```python
from build123d import *

# Parameters (mm, degrees)
SKETCH1_R           = 4
SKETCH1_R_2         = 2.5
BOSS_EXTRUDE1_DEPTH = 5
BOSS_EXTRUDE2_START = 3.5
SKETCH2_R           = 12.5
SKETCH2_R_2         = 2.5
BOSS_EXTRUDE2_DEPTH = 3.5
CIRPATTERN1_COUNT   = 4
CIRPATTERN2_COUNT   = 4
CHAMFER1_SIZE       = 0.5
SKETCH9_R           = 2.5
BOSS_EXTRUDE3_DEPTH = 2.9


with BuildPart() as part:
    # Sketch1 → Boss-Extrude1 (new body)
    with BuildSketch(Plane.XY):
        Circle(SKETCH1_R)
        Circle(SKETCH1_R_2, mode=Mode.SUBTRACT)
    extrude(amount=-BOSS_EXTRUDE1_DEPTH)

    # Sketch2 → Boss-Extrude2 (add)
    with BuildSketch(Plane.XY.offset(BOSS_EXTRUDE2_START)):
        Circle(SKETCH2_R)
        Circle(SKETCH2_R_2, mode=Mode.SUBTRACT)
    extrude(amount=-BOSS_EXTRUDE2_DEPTH)

    # Sketch6 → Tap Drill for M3 Tap1 (revolve, cut)
    with BuildSketch(Plane(origin=(4, 0, -2.5), x_dir=(0, 0, -1), z_dir=(0, 1, 0))):
        Polygon((0, 0), (0, 5.751075774), (1.25, 5), (1.25, 0.025), (1.275, 0), align=None)
    tap_drill_for_m3_tap1 = revolve(axis=Axis((10.35, 0, -2.5), (-1, 0, 0)), mode=Mode.SUBTRACT)

    # Sketch8 → Tap Drill for M3 Tap2 (revolve, cut)
    with BuildSketch(Plane(origin=(-9, 0, 3.5), x_dir=(0, -1, 0), z_dir=(1, 0, 0))):
        Polygon((0, 0), (0, 5.751075774), (1.25, 5), (1.25, 0.025), (1.275, 0), align=None)
    tap_drill_for_m3_tap2 = revolve(axis=Axis((-9, 0, 9.85), (0, 0, -1)), mode=Mode.SUBTRACT)

    # CirPattern1: Tap Drill for M3 Tap2 ×4 about axis
    cirpattern1_axis = Axis((0, 0, 0), (0, 0, 1))
    for i in range(1, CIRPATTERN1_COUNT):
        add(tap_drill_for_m3_tap2.rotate(cirpattern1_axis, i * 360 / CIRPATTERN1_COUNT), mode=Mode.SUBTRACT)

    # CirPattern2: Tap Drill for M3 Tap1 ×4 about axis
    cirpattern2_axis = Axis((0, 0, 0), (0, 0, 1))
    for i in range(1, CIRPATTERN2_COUNT):
        add(tap_drill_for_m3_tap1.rotate(cirpattern2_axis, i * 360 / CIRPATTERN2_COUNT), mode=Mode.SUBTRACT)

    # Chamfer1
    chamfer1_edges = [part.edges().sort_by_distance(p)[0] for p in [
        (-4, 0, -5),
    ]]
    chamfer(chamfer1_edges, length=CHAMFER1_SIZE)

    # Sketch9 → Boss-Extrude3 (add)
    with BuildSketch(Plane.XY.offset(3.5)):
        Circle(SKETCH9_R)
    extrude(amount=-BOSS_EXTRUDE3_DEPTH)


solid = part.part
```
The listing builds one solid part. Answer for the finished solid, in the listing's coordinates (mm). A direction names the side the tool comes from. Round coordinates to 2 decimals unless told otherwise and drop trailing zeros. Loops run counter-clockwise (first coordinate to the right, second up) from the corner with the lowest first, then second, coordinate; pieces in that order, holes last. Notation, with made-up numbers: (86.25, -2) -> (140.25, -2) arc R28 cw to (140.25, 34) -> close; hole circle Ø4 at (-36, 68.5). An arc over 180 degrees is marked (long way). Use one line per item in the form item = value.
1. A tool of negligible diameter and unlimited length cuts with its end or side. For faces 1 (the cylindrical face through (-3.08, 0.38, -3.69)), 2 (the flat face through (-3, 3, 0)), from which of +Z, -Z, +X, -X, +Y, -Y can it reach the whole face along a straight path? Write none if from no direction.
Answer key:
face_1 = +X, -X
face_2 = -Z
2. Flat-ended cylindrical pins translate along their axes: pin 1 Ø3 at (x, z) = (0, -2.5) entering from +Y; pin 2 Ø4 at (x, y) = (9, 0) entering from -Z; pin 3 Ø1.5 at (y, z) = (-4, 2) entering from +X. Find the tip coordinate at first contact, or state that the pin passes through.
Answer key:
pin_1 = 4
pin_2 = 0
pin_3 = 12.07
3. Find the intervals of material crossed by probe 1 along Y at (x, z) = (0, 2.8); probe 2 along Z at (x, y) = (0, -2.6); probe 3 along Z at (x, y) = (2, 8.5), in increasing order. Write a range as [from, to].
Answer key:
probe_1 = [-12.5, -10.25], [-7.75, 7.75], [10.25, 12.5]
probe_2 = [-5, -3.75], [-1.25, 3.5]
probe_3 = [0, 3.5]
4. The part is cut by section B-B on z = -2.5. Determine the outline of the cut face in (x, y), and give its area (3 significant figures).
Answer key:
outline = (-3.8, -1.25) arc R4 ccw to (-1.25, -3.8) -> (-1.25, -2.17) arc R2.5 cw to (-2.17, -1.25) -> close; (-3.8, 1.25) -> (-2.17, 1.25) arc R2.5 cw to (-1.25, 2.17) -> (-1.25, 3.8) arc R4 ccw to start; (1.25, -3.8) arc R4 ccw to (3.8, -1.25) -> (2.17, -1.25) arc R2.5 cw to (1.25, -2.17) -> close; (1.25, 2.17) arc R2.5 cw to (2.17, 1.25) -> (3.8, 1.25) arc R4 ccw to (1.25, 3.8) -> close
area = 15.2 mm²
5. For a pull along X with two mould halves and no side action, classify faces 3 (the cylindrical face through (-1.84, 1.69, -2.16)), 4 (the cylindrical face through (3.695, -1.532, -2.218)), 5 (the flat face through (2, -2, -5)) as released by +X, released by -X, zero draft, split by the parting line, or undercut.
Answer key:
face_3 = undercut
face_4 = split by the parting line
face_5 = zero draft
6. The part is cut by section A-A on y = 9. Determine the outline of the cut face in (x, z) (3 decimals), and give its area (3 significant figures).
Answer key:
outline = (-8.675, 0) -> (-1.25, 0) -> (-1.25, 3.475) -> (-1.275, 3.5) -> (-8.675, 3.5) -> close; (1.25, 0) -> (8.675, 0) -> (8.675, 3.5) -> (1.275, 3.5) -> (1.25, 3.475) -> close
area = 52.0 mm²
7. The part is cut by section D-D on z = 1.5. Determine the outline of the cut face in (x, y), and give its area (3 significant figures).
Answer key:
outline = circle Ø25 at (0, 0); hole circle Ø2.5 at (-9, 0); hole circle Ø2.5 at (0, -9); hole circle Ø2.5 at (0, 9); hole circle Ø2.5 at (9, 0)
area = 471 mm²
